Input: part model. Units: mm. Frame: model coordinates. A direction names the side the tool comes from. Give positions to 0.01 mm unless a question says otherwise; leave off trailing zeros. Order: outer loops, then holes, each group sorted by start corner. A loop starts at its lowest first (then second) coordinate and runs counter-clockwise, first axis right, second up.
Solid Edge part; units mm, degrees
sketch "Sketch1" plane through (0, 0, 0) normal (0, 0, 1) x (1, 0, 0)
  circle A0 centre (92.5, 80) radius 2
  circle A1 centre (-92.5, 80) radius 2
  circle A2 centre (-92.5, -80) radius 2
  arc A3 (-48, -25.0015) -> (-47, -26.0015) centre (-48, -26.0015) cw
  line L0 (-47, -26.0015) -> (-47, -70.0015)
  arc A4 (-47, -70.0015) -> (-48, -71.0015) centre (-48, -70.0015) cw
  line L1 (-48, -71.0015) -> (-75, -71.0015)
  arc A5 (-75, -71.0015) -> (-76, -70.0015) centre (-75, -70.0015) cw
  line L2 (-76, -70.0015) -> (-76, -26.0015)
  arc A6 (-76, -26.0015) -> (-75, -25.0015) centre (-75, -26.0015) cw
  line L3 (-75, -25.0015) -> (-48, -25.0015)
  arc A7 (-7, -25.0015) -> (-6, -26.0015) centre (-7, -26.0015) cw
  line L4 (-6, -26.0015) -> (-6, -70.0015)
  arc A8 (-6, -70.0015) -> (-7, -71.0015) centre (-7, -70.0015) cw
  line L5 (-7, -71.0015) -> (-34, -71.0015)
  arc A9 (-34, -71.0015) -> (-35, -70.0015) centre (-34, -70.0015) cw
  line L6 (-35, -70.0015) -> (-35, -26.0015)
  arc A10 (-35, -26.0015) -> (-34, -25.0015) centre (-34, -26.0015) cw
  line L7 (-34, -25.0015) -> (-7, -25.0015)
  arc A11 (34, -25.0015) -> (35, -26.0015) centre (34, -26.0015) cw
  line L8 (35, -26.0015) -> (35, -70.0015)
  arc A12 (35, -70.0015) -> (34, -71.0015) centre (34, -70.0015) cw
  line L9 (34, -71.0015) -> (7, -71.0015)
  arc A13 (7, -71.0015) -> (6, -70.0015) centre (7, -70.0015) cw
  line L10 (6, -70.0015) -> (6, -26.0015)
  arc A14 (6, -26.0015) -> (7, -25.0015) centre (7, -26.0015) cw
  line L11 (7, -25.0015) -> (34, -25.0015)
  arc A15 (75, -25.0015) -> (76, -26.0015) centre (75, -26.0015) cw
  line L12 (76, -26.0015) -> (76, -70.0015)
  arc A16 (76, -70.0015) -> (75, -71.0015) centre (75, -70.0015) cw
  line L13 (75, -71.0015) -> (48, -71.0015)
  arc A17 (48, -71.0015) -> (47, -70.0015) centre (48, -70.0015) cw
  line L14 (47, -70.0015) -> (47, -26.0015)
  arc A18 (47, -26.0015) -> (48, -25.0015) centre (48, -26.0015) cw
  line L15 (48, -25.0015) -> (75, -25.0015)
  arc A19 (54.5, 30.9985) -> (55.5, 29.9985) centre (54.5, 29.9985) cw
  line L16 (55.5, 29.9985) -> (55.5, -14.0015)
  arc A20 (55.5, -14.0015) -> (54.5, -15.0015) centre (54.5, -14.0015) cw
  line L17 (54.5, -15.0015) -> (27.5, -15.0015)
  arc A21 (27.5, -15.0015) -> (26.5, -14.0015) centre (27.5, -14.0015) cw
  line L18 (26.5, -14.0015) -> (26.5, 29.9985)
  arc A22 (26.5, 29.9985) -> (27.5, 30.9985) centre (27.5, 29.9985) cw
  line L19 (27.5, 30.9985) -> (54.5, 30.9985)
  arc A23 (13.5, 30.9985) -> (14.5, 29.9985) centre (13.5, 29.9985) cw
  line L20 (14.5, 29.9985) -> (14.5, -14.0015)
  arc A24 (14.5, -14.0015) -> (13.5, -15.0015) centre (13.5, -14.0015) cw
  line L21 (13.5, -15.0015) -> (-13.5, -15.0015)
  arc A25 (-13.5, -15.0015) -> (-14.5, -14.0015) centre (-13.5, -14.0015) cw
  line L22 (-14.5, -14.0015) -> (-14.5, 29.9985)
  arc A26 (-14.5, 29.9985) -> (-13.5, 30.9985) centre (-13.5, 29.9985) cw
  line L23 (-13.5, 30.9985) -> (13.5, 30.9985)
  arc A27 (69, 74.9985) -> (70, 73.9985) centre (69, 73.9985) cw
  line L24 (70, 73.9985) -> (70, 46.9985)
  arc A28 (70, 46.9985) -> (69, 45.9985) centre (69, 46.9985) cw
  line L25 (69, 45.9985) -> (42, 45.9985)
  arc A29 (42, 45.9985) -> (41, 46.9985) centre (42, 46.9985) cw
  line L26 (41, 46.9985) -> (41, 73.9985)
  arc A30 (41, 73.9985) -> (42, 74.9985) centre (42, 73.9985) cw
  line L27 (42, 74.9985) -> (69, 74.9985)
  arc A31 (96.5, 90) -> (102.5, 84) centre (96.5, 84) cw
  line L28 (102.5, 84) -> (102.5, -84)
  arc A32 (102.5, -84) -> (96.5, -90) centre (96.5, -84) cw
  line L29 (96.5, -90) -> (-96.5, -90)
  arc A33 (-96.5, -90) -> (-102.5, -84) centre (-96.5, -84) cw
  line L30 (-102.5, -84) -> (-102.5, 84)
  arc A34 (-102.5, 84) -> (-96.5, 90) centre (-96.5, 84) cw
  line L31 (-96.5, 90) -> (96.5, 90)
  arc A35 (-42, 74.9985) -> (-41, 73.9985) centre (-42, 73.9985) cw
  line L32 (-41, 73.9985) -> (-41, 46.9985)
  arc A36 (-41, 46.9985) -> (-42, 45.9985) centre (-42, 46.9985) cw
  line L33 (-42, 45.9985) -> (-69, 45.9985)
  arc A37 (-69, 45.9985) -> (-70, 46.9985) centre (-69, 46.9985) cw
  line L34 (-70, 46.9985) -> (-70, 73.9985)
  arc A38 (-70, 73.9985) -> (-69, 74.9985) centre (-69, 73.9985) cw
  line L35 (-69, 74.9985) -> (-42, 74.9985)
  arc A39 (-27.5, 30.9985) -> (-26.5, 29.9985) centre (-27.5, 29.9985) cw
  line L36 (-26.5, 29.9985) -> (-26.5, -14.0015)
  arc A40 (-26.5, -14.0015) -> (-27.5, -15.0015) centre (-27.5, -14.0015) cw
  line L37 (-27.5, -15.0015) -> (-54.5, -15.0015)
  arc A41 (-54.5, -15.0015) -> (-55.5, -14.0015) centre (-54.5, -14.0015) cw
  line L38 (-55.5, -14.0015) -> (-55.5, 29.9985)
  arc A42 (-55.5, 29.9985) -> (-54.5, 30.9985) centre (-54.5, 29.9985) cw
  line L39 (-54.5, 30.9985) -> (-27.5, 30.9985)
  circle A43 centre (92.5, -80) radius 2
  dimension "D1" = 92.5
  dimension "D2" = 92.5
extrude "Protrusion1" add sketch "Sketch1" along normal blind 5
1) Cut plane D-D (y = -50.5). Return the cut outline in (x, z).
2) Cut plane A-A (y = 53). Return the cut outline in (x, z), then the cut area to 3 significant figures.
3) Reachability of faces 4 (the face through (-100.696, -88.289, 2.465)), 5 (the face through (0, -15.002, 2)) from +Z, -Z, +X, -X, +Y, -Y: full face, straight path, thin tool, end or side. Return the list, or none.
4) Pull-direction query (Y, two-part tool) for faces 1 (the face through (-100.789, 88.196, 2.465)), 2 (the face through (-55, 45.998, 2)), 3 (the face through (-21, 1, 0)); classes: pulls with the +Y half, pulls with the -Y half, needs draft (parallel to the pull), parting line crosses it, or undercut.
5) Cut plane C-C (x = 51.5). Return the cut outline in (y, z).
6) Cut plane B-B (x = -17). Return the cut outline in (y, z), then the cut area to 3 significant figures.
7) Line query: probe 1 along X at (y, z) = (-12, 3.25); probe 2 along Y at (x, z) = (-9, 1.3); probe 3 along X at (y, z) = (49, 1.7). Output: solid intervals per line, ascending.
Geometry says:
1. outline: (-102.5, 0) - (-76, 0) - (-76, 5) - (-102.5, 5) - close; (-47, 0) - (-35, 0) - (-35, 5) - (-47, 5) - close; (-6, 0) - (6, 0) - (6, 5) - (-6, 5) - close; (35, 0) - (47, 0) - (47, 5) - (35, 5) - close; (76, 0) - (102.5, 0) - (102.5, 5) - (76, 5) - close
2. outline: (-102.5, 0) - (-70, 0) - (-70, 5) - (-102.5, 5) - close; (-41, 0) - (41, 0) - (41, 5) - (-41, 5) - close; (70, 0) - (102.5, 0) - (102.5, 5) - (70, 5) - close
2. area: 735 mm2
3. face 4: +Z, -Z, -X, -Y
3. face 5: +Z, -Z
4. face 1: pulls with the +Y half
4. face 2: undercut
4. face 3: needs draft
5. outline: (-90, 0) - (-71, 0) - (-71, 5) - (-90, 5) - close; (-25, 0) - (-15, 0) - (-15, 5) - (-25, 5) - close; (31, 0) - (46, 0) - (46, 5) - (31, 5) - close; (75, 0) - (90, 0) - (90, 5) - (75, 5) - close
6. outline: (-90, 0) - (-71, 0) - (-71, 5) - (-90, 5) - close; (-25, 0) - (90, 0) - (90, 5) - (-25, 5) - close
6. area: 670 mm2
7. probe 1: x = -102.5 to -55.5, -26.5 to -14.5, 14.5 to 26.5, 55.5 to 102.5
7. probe 2: y = -90 to -71, -25 to -15, 31 to 90
7. probe 3: x = -102.5 to -70, -41 to 41, 70 to 102.5
